from build123d import *

# Parameters (mm, degrees)
BOSS_EXTRUDE1_START         = 4.5
SKETCH2_W                   = 231.966777064
SKETCH2_H                   = 36.14
BOSS_EXTRUDE1_DEPTH         = 2
SKETCH3_R                   = 3.5
BOSS_EXTRUDE2_DEPTH         = 4.5
TAP_DRILL_FOR_M3X0_5_TAP1_D = 2.5


with BuildPart() as part:
    # Sketch2 → Boss-Extrude1 (new body)
    with BuildSketch(Plane(origin=(0, 0, -1.6), x_dir=(-1, 0, 0), z_dir=(0, 0, -1)).offset(BOSS_EXTRUDE1_START)):
        with Locations((-174.403388532, -55.59)):
            Rectangle(SKETCH2_W, SKETCH2_H)
    extrude(amount=BOSS_EXTRUDE1_DEPTH)

    # Sketch3 → Boss-Extrude2 (add)
    with BuildSketch(Plane.XY.offset(-6.1)):
        with Locations(Location((271.78, -45.72, 0), (0, 0, 180))):
            Circle(SKETCH3_R)
        with Locations(Location((271.78, -68.58, 0), (0, 0, 180))):
            Circle(SKETCH3_R)
        with Locations(Location((214.63, -52.07, 0), (0, 0, 180))):
            Circle(SKETCH3_R)
        with Locations(Location((76.2, -45.72, 0), (0, 0, 180))):
            Circle(SKETCH3_R)
        with Locations(Location((76.2, -68.58, 0), (0, 0, 180))):
            Circle(SKETCH3_R)
    extrude(amount=BOSS_EXTRUDE2_DEPTH)

    # Tap Drill for M3x0.5 Tap1 (through all)
    with Locations(Plane.XY.offset(-1.6)):
        with Locations((271.78, -45.72), (271.78, -68.58), (214.63, -52.07), (76.2, -45.72), (76.2, -68.58)):
            Hole(TAP_DRILL_FOR_M3X0_5_TAP1_D / 2)


solid = part.part
Can you work these out from the model? Positions are in its coordinate system, mm. A direction names the side the tool comes from. Round coordinates to 2 decimals unless told otherwise and drop trailing zeros. Loops run counter-clockwise (first coordinate to the right, second up) from the corner with the lowest first, then second, coordinate; pieces in that order, holes last. Notation, with made-up numbers: (-7.75, 19.5) - (6.25, 19.5) arc R21 cw to (6.25, 58.5) - close; hole circle Ø8 at (62.5, -21.75). An arc over 180 degrees is marked (long way). Answer in a Markdown table with one row per item. Add a question column.
Q1. For pin 1 Ø1.5 at (x, y) = (126, -56.5) entering from +Z; pin 2 Ø2 at (x, z) = (190, -4) entering from -Y, each with a flat end and sliding along its axis, tell me the tip position at first contact or that it passes through.
Q2. Which directions (+Z, -Z, +X, -X, +Y, -Y) give clear straight access to the entire face, cutting with the end or side of a thin tool? Please do faces 1 (the flat face through (76, -67, -1.6)), 2 (the cylindrical face through (268.44, -46.77, -3.88)).
Q3. We'd pull the mould along Y, two halves only. Please class faces 3 (the cylindrical face through (79.697, -45.874, -3.881)), 4 (the cylindrical face through (268.44, -69.63, -3.88)), 5 (the cylindrical face through (217.407, -49.94, -3.881)), 6 (the flat face through (270, -69, -1.6)): pulls with the +Y half, pulls with the -Y half, needs draft (parallel to the pull), parting line crosses it, or undercut.
Q4. I need wall thicknesses on L1, parallel to Y at x = 271.78, z = -3.5; L2, parallel to X at y = -68.58, z = -5; L3, parallel to X at y = -45, z = -6. Which ranges of each line are inside material? Lowest first, please.
Q5. I want a section at A-A on y = -58. List the corners of the cut face in (x, z) for me, and give its area (3 significant figures).
Q6. I want a section at B-B on x = 87. List the corners of the cut face in (y, z) for me.
A:
| question | item | result |
|---|---|---|
| 1 | pin 1 | z = -6.1 |
| 1 | pin 2 | through |
| 2 | face 1 | +Z, +X, -X, +Y, -Y |
| 2 | face 2 | +Z |
| 3 | face 3 | undercut |
| 3 | face 4 | undercut |
| 3 | face 5 | parting line crosses it |
| 3 | face 6 | needs draft |
| 4 | L1 | -72.08 to -69.83, -67.33 to -65.08, -49.22 to -46.97, -44.47 to -42.22 |
| 4 | L2 | 72.7 to 74.95, 77.45 to 79.7, 268.28 to 270.53, 273.03 to 275.28 |
| 4 | L3 | 72.77 to 75.18, 77.22 to 79.63, 268.35 to 270.76, 272.8 to 275.21 |
| 5 | outline | (58.42, -8.1) - (290.39, -8.1) - (290.39, -6.1) - (58.42, -6.1) - close |
| 5 | area | 464 mm^2 |
| 6 | outline | (-73.66, -8.1) - (-37.52, -8.1) - (-37.52, -6.1) - (-73.66, -6.1) - close |
